Here's how the part is built. I have some questions about the finished solid (model axes, mm). Round coordinates to 2 decimals unless told otherwise and drop trailing zeros. Write each loop counter-clockwise with the first axis right and the second up, starting at its lowest first coordinate (ties: lowest second). Pieces come first, ordered by that corner, then holes. Notation, with made-up numbers: (26, 19) - (37, 19) arc R14 cw to (37, 35) - close; hole circle Ø8 at (12.25, 9). An arc over 180 degrees is marked (long way). Write item = value, one per line. Start each with the question number.
Item 1: If I drill on line 1 along X through (y, z) = (5, 0); line 2 along X through (y, z) = (2.75, 8), over which ranges is the centre line in solid material (lowest first)? Write a range as [from, to].
Item 2: If we section it at A-A (x = -8): Please give me the cut outline in (y, z).
Item 3: Thinking about a two-plate mould opening in X: for faces 1 (the face through (-9.5, 5.07, -0.07)), 2 (the face through (0, 5, 25)), 3 (the face through (25, 5, 0)), 4 (the face through (2.4, 5.1, 4.5)), which applies, pulls with the +X half, pulls with the -X half, needs draft (parallel to the pull), parting line crosses it, or undercut?
Item 4: If we section it at B-B (z = 0): Please give me the cut outline in (x, y).
Item 5: If we section it at C-C (y = 9): Please give me the cut outline in (x, z), and give its area (3 significant figures).
Item 6: If we section it at D-D (x = 0): Please give me the cut outline in (y, z), and give its area (3 significant figures).
Autodesk Inventor part; units mm, degrees
ref_plane "YZ Plane" through (0, 0, 0) normal (1, 0, 0) x (0, 1, 0)
ref_plane "XZ Plane" through (0, 0, 0) normal (0, 1, 0) x (-1, 0, 0)
ref_plane "XY Plane" through (0, 0, 0) normal (0, 0, 1) x (1, 0, 0)
sketch "Sketch1" plane through (0, 0, 0) normal (0, 1, 0) x (-1, 0, 0)
  line L0 (25, -25) -> (-25, -25)
  line L1 (-25, -25) -> (-25, 25)
  line L2 (-25, 25) -> (25, 25)
  line L3 (25, 25) -> (25, -25)
  line L4 (25, -25) -> (-25, 25) construction
  line L5 (-25, -25) -> (25, 25) construction
  point P0 (0, 0)
  dimension "d0" = 50
  dimension "d1" = 50
extrude "Extrusion1" add sketch "Sketch1" along normal blind 10
sketch "Sketch2" plane through (0, 10, 0) normal (0, 1, 0) x (1, 0, 0)
  line L0 (25, -25) -> (25, 25)
  line L1 (0, 0) -> (0, 8)
  circle A0 centre (0, 8) radius 1.5
  circle A1 centre (0, 0) radius 5.1
  circle A2 centre (-8, 0) radius 1.5
  circle A3 centre (0, -8) radius 1.5
  circle A4 centre (8, 0) radius 1.5
  dimension "d4" = 8
  dimension "screw_hole" = 3
  dimension "center_hole" = 10.2
  dimension "d9" = 360
extrude "Extrusion2" cut sketch "Sketch2" against normal up to next
properties part number "ACMENUTgen"
Reply:
q1.line_1 = [-25, -9.5], [-6.5, -5.1], [5.1, 6.5], [9.5, 25]
q1.line_2 = [-25, -1.5], [1.5, 25]
q2.outline = (0, -25) - (10, -25) - (10, -1.5) - (0, -1.5) - close; (0, 1.5) - (10, 1.5) - (10, 25) - (0, 25) - close
q3.face_1 = undercut
q3.face_2 = needs draft
q3.face_3 = pulls with the +X half
q3.face_4 = undercut
q4.outline = (-25, 0) - (-9.5, 0) - (-9.5, 10) - (-25, 10) - close; (-6.5, 0) - (-5.1, 0) - (-5.1, 10) - (-6.5, 10) - close; (5.1, 0) - (6.5, 0) - (6.5, 10) - (5.1, 10) - close; (9.5, 0) - (25, 0) - (25, 10) - (9.5, 10) - close
q5.outline = (-25, -25) - (25, -25) - (25, 25) - (-25, 25) - close; hole circle Ø3 at (-8, 0); hole circle Ø10.2 at (0, 0); hole circle Ø3 at (0, -8); hole circle Ø3 at (0, 8); hole circle Ø3 at (8, 0)
q5.area = 2,390 mm2
q6.outline = (0, -25) - (10, -25) - (10, -9.5) - (0, -9.5) - close; (0, -6.5) - (10, -6.5) - (10, -5.1) - (0, -5.1) - close; (0, 5.1) - (10, 5.1) - (10, 6.5) - (0, 6.5) - close; (0, 9.5) - (10, 9.5) - (10, 25) - (0, 25) - close
q6.area = 338 mm2
